from build123d import *

# Parameters (mm, degrees)
ESQUISSE1_W             = 54
ESQUISSE1_H             = 54
BOSS_EXTRU_1_DEPTH      = 67.37
ESQUISSE2_W             = 85.887974464
ESQUISSE2_H             = 58.790343592
ENL_V_MAT_EXTRU_1_DEPTH = 62.37
ESQUISSE3_R             = 3
ENL_V_MAT_EXTRU_2_DEPTH = 62.37
D_GAGEMENT_M61_D        = 6.6


with BuildPart() as part:
    # Esquisse1 → Boss.-Extru.1 (new body)
    with BuildSketch(Plane.XY):
        Rectangle(ESQUISSE1_W, ESQUISSE1_H)
    extrude(amount=BOSS_EXTRU_1_DEPTH)

    # Esquisse2 → Enlèv. mat.-Extru.1 (cut)
    with BuildSketch(Plane.XY.offset(67.37)):
        with Locations((-4.168944697, -6.395171796)):
            Rectangle(ESQUISSE2_W, ESQUISSE2_H)
    extrude(amount=-ENL_V_MAT_EXTRU_1_DEPTH, mode=Mode.SUBTRACT)

    # Esquisse3 → Enlèv. mat.-Extru.2 (cut)
    with BuildSketch(Plane.XZ.offset(-23)):
        with Locations(Location((-20, 59.37, 0), (0, 0, 270))):
            Circle(ESQUISSE3_R)
        with Locations(Location((20, 59.37, 0), (0, 0, 270))):
            Circle(ESQUISSE3_R)
    extrude(amount=-ENL_V_MAT_EXTRU_2_DEPTH, mode=Mode.SUBTRACT)

    # Dégagement M61 (through all)
    with Locations(Plane(origin=(0, 0, 0), x_dir=(-1, 0, 0), z_dir=(0, 0, -1))):
        with Locations((20.562817304, -15.5), (20.562817304, 16.5)):
            Hole(D_GAGEMENT_M61_D / 2)


solid = part.part
Design review of the part built by this model. Coordinates are the model's own, in mm. A direction names the side the tool comes from. Round coordinates to 2 decimals unless told otherwise and drop trailing zeros. Loops run counter-clockwise (first coordinate to the right, second up) from the corner with the lowest first, then second, coordinate; pieces in that order, holes last. Notation, with made-up numbers: (24.5, -28.75) - (51.5, -28.75) arc R17 ccw to (51.5, 2.25) - close; hole circle Ø9 at (-17.5, 61). An arc over 180 degrees is marked (long way). One line per question, with ' | ' between items.
1. We need section A-A, the plane x = 20. State the section outline as (y, z) points, and give its area (3 significant figures).
Results are:
outline: (-27, 0) - (27, 0) - (27, 56.37) - (23, 56.37) - (23, 5) - (-27, 5) - close; (23, 62.37) - (27, 62.37) - (27, 67.37) - (23, 67.37) - close | area: 495 mm²
2. We need section D-D, the plane x = -20. State the section outline as (y, z) points.
Results are:
outline: (-27, 0) - (-18.75, 0) - (-18.75, 5) - (-27, 5) - close; (-12.25, 0) - (13.25, 0) - (13.25, 5) - (-12.25, 5) - close; (19.75, 0) - (27, 0) - (27, 56.37) - (23, 56.37) - (23, 5) - (19.75, 5) - close; (23, 62.37) - (27, 62.37) - (27, 67.37) - (23, 67.37) - close
3. We need section C-C, the plane z = 59.37. State the section outline as (x, y) points.
Results are:
outline: (-27, 23) - (-23, 23) - (-23, 27) - (-27, 27) - close; (-17, 23) - (17, 23) - (17, 27) - (-17, 27) - close; (23, 23) - (27, 23) - (27, 27) - (23, 27) - close
4. Draft analysis for pull direction X (two halves, no side actions). For faces 3 (the face through (-19.868, 24.972, 62.367)), 4 (the face through (0, 25, 67.37)), 5 (the face through (-27, 24, 19)), state which applies: released by +X, released by -X, zero draft, split by the parting line, or undercut.
Results are:
face 3: undercut | face 4: zero draft | face 5: released by -X
5. For faces 1 (the face through (0, 23, 37)), 2 (the face through (0, 27, 33)), list the 3-axis set-ups (+Z, -Z, +X, -X, +Y, -Y) from which the entire face can be reached by the end or side of a thin tool; tool diameter is ignored.
Results are:
face 1: +Z, +X, -X, -Y | face 2: +Z, -Z, +X, -X, +Y
6. For L1, parallel to X at y = 25.5, z = 59.37; L2, parallel to Y at x = 8, z = 54; L3, parallel to Z at x = 9.5, y = -22, list the stretches that pass through material, from the lowest coordinate up. Write a range as [from, to].
Results are:
L1: x = [-27, -23], [-17, 17], [23, 27] | L2: y = [23, 27] | L3: z = [0, 5]
7. We need section B-B, the plane y = 16.5. State the section outline as (x, z) points, and give its area (3 significant figures).
Results are:
outline: (-27, 0) - (-23.86, 0) - (-23.86, 5) - (-27, 5) - close; (-17.26, 0) - (27, 0) - (27, 5) - (-17.26, 5) - close | area: 237 mm²
8. Clearance check with flat-ended pins moving along their axes: P1, Ø10, axis at x = 6, z = 32.5, coming from the -Y side; P2, Ø1.5, axis at y = 20.5, z = 52.5, coming from the -X side; P3, Ø1, axis at x = -2, y = 11, coming from the +Z side. State where each tip first meets the part, or that it passes through.
Results are:
P1: stops at y = 23 | P2: passes through | P3: stops at z = 5
